from build123d import *

# Parameters (mm, degrees)
F0_R     = 0.635
F1_DEPTH = 2.54
F2_R     = 1.26999


# Not quite as in the source:
# - a fillet or chamfer is up to 0.001 mm smaller than in the source, because OpenCascade refuses the exact size


with BuildPart() as f1:
    # F0 (on Front) → F1 (new body)
    with BuildSketch(Plane.XZ):
        Polygon((15.0977487051, 33.894000689), (-8.7011743405, 33.894000689), (-8.7011743405, 30.6449289119), (-8.7011743405, 30.6394077664), (-8.7011743405, 28.5887729555), (-8.7011743405, 28.1049289119), (-8.7011743405, 23.0249289119), (21.375445649, 23.0249289119), (37.1712256595, 23.0249289119), (37.1712256595, 27.0205680281), (38.9492256595, 27.0205680281), (38.9492256595, 30.7752811804), (38.9492256595, 33.6518122062), (17.204430995, 33.6518122062), (17.204430995, 30.7752811804), (15.0977487051, 30.7752811804), align=None)
        with BuildLine():
            ThreePointArc((-6.7956986329, 25.5649289119), (-6.9816858268, 25.1159161058), (-7.4306986329, 24.9299289119))
            ThreePointArc((-7.4306986329, 24.9299289119), (-7.8797114389, 25.1159161058), (-8.0656986329, 25.5649289119))
            ThreePointArc((-8.0656986329, 25.5649289119), (-7.8797114389, 26.0139417179), (-7.4306986329, 26.1999289119))
            ThreePointArc((-7.4306986329, 26.1999289119), (-6.9816858268, 26.0139417179), (-6.7956986329, 25.5649289119))
        make_face(mode=Mode.SUBTRACT)
        with BuildLine():
            ThreePointArc((-7.4306986329, 28.7399289119), (-6.9816858268, 28.5539417179), (-6.7956986329, 28.1049289119))
            ThreePointArc((-6.7956986329, 28.1049289119), (-6.9816858268, 27.6559161058), (-7.4306986329, 27.4699289119))
            ThreePointArc((-7.4306986329, 27.4699289119), (-7.8797114389, 27.6559161058), (-8.0656986329, 28.1049289119))
            ThreePointArc((-8.0656986329, 28.1049289119), (-7.8797114389, 28.5539417179), (-7.4306986329, 28.7399289119))
        make_face(mode=Mode.SUBTRACT)
        with BuildLine():
            ThreePointArc((-7.4306986329, 30.0099289119), (-7.8797114389, 30.1959161058), (-8.0656986329, 30.6449289119))
            ThreePointArc((-8.0656986329, 30.6449289119), (-7.8797114389, 31.0939417179), (-7.4306986329, 31.2799289119))
            ThreePointArc((-7.4306986329, 31.2799289119), (-6.9816858268, 31.0939417179), (-6.7956986329, 30.6449289119))
            ThreePointArc((-6.7956986329, 30.6449289119), (-6.9816858268, 30.1959161058), (-7.4306986329, 30.0099289119))
        make_face(mode=Mode.SUBTRACT)
        with BuildLine():
            ThreePointArc((13.1927487051, 25.5649289119), (13.0067615112, 25.1159161058), (12.5577487051, 24.9299289119))
            ThreePointArc((12.5577487051, 24.9299289119), (11.9227487051, 25.5649289119), (12.5577487051, 26.1999289119))
            ThreePointArc((12.5577487051, 26.1999289119), (13.0067615112, 26.0139417179), (13.1927487051, 25.5649289119))
        make_face(mode=Mode.SUBTRACT)
        with BuildLine():
            ThreePointArc((12.5577487051, 28.7399289119), (13.0067615112, 28.5539417179), (13.1927487051, 28.1049289119))
            ThreePointArc((13.1927487051, 28.1049289119), (13.0067615112, 27.6559161058), (12.5577487051, 27.4699289119))
            ThreePointArc((12.5577487051, 27.4699289119), (11.9227487051, 28.1049289119), (12.5577487051, 28.7399289119))
        make_face(mode=Mode.SUBTRACT)
        with BuildLine():
            ThreePointArc((13.1927487051, 30.6449289119), (13.0067615112, 30.1959161058), (12.5577487051, 30.0099289119))
            ThreePointArc((12.5577487051, 30.0099289119), (11.9227487051, 30.6449289119), (12.5577487051, 31.2799289119))
            ThreePointArc((12.5577487051, 31.2799289119), (13.0067615112, 31.0939417179), (13.1927487051, 30.6449289119))
        make_face(mode=Mode.SUBTRACT)
        with Locations((19.744430995, 25.3227458062)):
            Circle(F0_R, mode=Mode.SUBTRACT)
        with Locations((19.744430995, 27.8627458062)):
            Circle(F0_R, mode=Mode.SUBTRACT)
        with Locations((19.744430995, 30.4027458062)):
            Circle(F0_R, mode=Mode.SUBTRACT)
        with BuildLine():
            Line((21.375445649, 23.0249289119), (-8.7011743405, 23.0249289119))
            Line((-8.7011743405, 23.0249289119), (14.6481524707, 7.6804661495))
            Line((14.6481524707, 7.6804661495), (4.3133735196, -8.0457365195))
            Line((4.3133735196, -8.0457365195), (4.3133735196, -53.9590548808))
            Line((4.3133735196, -53.9590548808), (21.375445649, -53.9590548808))
            Line((21.375445649, -53.9590548808), (21.375445649, -19.4510648049))
            ThreePointArc((21.375445649, -19.4510648049), (20.105445649, -18.1810648049), (21.375445649, -16.9110648049))
            Line((21.375445649, -16.9110648049), (21.375445649, 23.0249289119))
        make_face()
        with BuildLine():
            Line((37.1712256595, 23.0249289119), (21.375445649, 23.0249289119))
            Line((21.375445649, 23.0249289119), (21.375445649, -16.9110648049))
            ThreePointArc((21.375445649, -16.9110648049), (22.2734712611, -17.2830391928), (22.645445649, -18.1810648049))
            Line((22.645445649, -18.1810648049), (30.3538220114, -18.1810648049))
            Line((30.3538220114, -18.1810648049), (30.3538220114, -7.9758184713))
            Line((30.3538220114, -7.9758184713), (38.9492256595, -7.9758184713))
            Line((38.9492256595, -7.9758184713), (38.9492256595, 5.319000689))
            Line((38.9492256595, 5.319000689), (38.9492256595, 21.9405680281))
            Line((38.9492256595, 21.9405680281), (37.1712256595, 21.9405680281))
            Line((37.1712256595, 21.9405680281), (37.1712256595, 23.0249289119))
        make_face()
        Polygon((4.3133735196, -53.9590548808), (4.3133735196, -8.0457365195), (-20.8784960799, -46.3796427219), (-44.3256125721, -31.185070223), (-46.598433602, -34.7022139158), (-30.3224786203, -45.2199339734), (-30.3224786203, -53.9590548808), align=None)
        with BuildLine():
            Line((30.3538220114, -18.1810648049), (22.645445649, -18.1810648049))
            ThreePointArc((22.645445649, -18.1810648049), (22.2734712611, -19.079090417), (21.375445649, -19.4510648049))
            Line((21.375445649, -19.4510648049), (21.375445649, -53.9590548808))
            Line((21.375445649, -53.9590548808), (38.9492256595, -53.9590548808))
            Line((38.9492256595, -53.9590548808), (38.9492256595, -45.480999311))
            Line((38.9492256595, -45.480999311), (38.9492256595, -42.0136552247))
            Line((38.9492256595, -42.0136552247), (37.1712256595, -42.0136552247))
            Line((37.1712256595, -42.0136552247), (37.1712256595, -36.9336552247))
            Line((37.1712256595, -36.9336552247), (38.9492256595, -36.9336552247))
            Line((38.9492256595, -36.9336552247), (38.9492256595, -28.3863111384))
            Line((38.9492256595, -28.3863111384), (30.3538220114, -28.3863111384))
            Line((30.3538220114, -28.3863111384), (30.3538220114, -18.1810648049))
        make_face()
        Polygon((38.9492256595, -42.0136552247), (38.9492256595, -45.480999311), (38.9764610146, -42.0136552247), align=None)
        Polygon((39.0835013158, -28.3863111384), (38.9492256595, -28.3863111384), (38.9492256595, -36.9336552247), (39.0163634877, -36.9336552247), align=None)
    extrude(amount=F1_DEPTH)

    # F2 (radius 1.27 in the source; OpenCascade refuses exactly that, so slightly less here)
    f2_edges = [f1.edges().sort_by_distance(p)[0] for p in [
        (20.105446, -2.54, -18.181065),
        (20.105446, 0, -18.181065),
    ]]
    fillet(f2_edges, radius=F2_R)


solid = f1.part
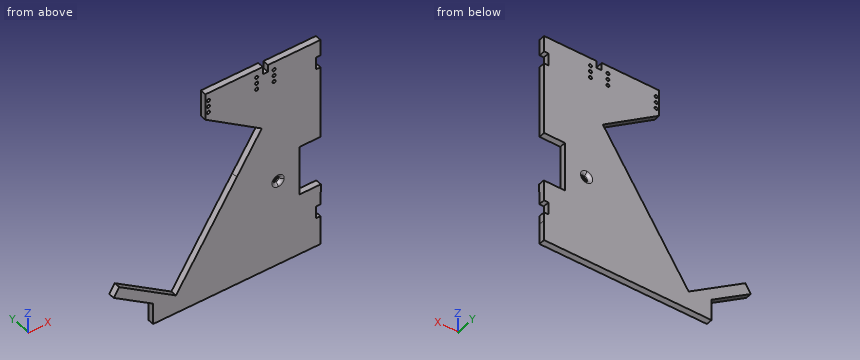
Part model, mm, in its own coordinate system. Coordinates: 2 decimals unless noted, no trailing zeros. Order: outer loops, then holes, each group sorted by start corner. A loop starts at its lowest first (then second) coordinate and runs counter-clockwise, first axis right, second up. Notation, with made-up numbers: M 44.25,3.5 L 103.25,3.5 A33 cw 103.25,36.5 Z; hole C -40,-15 d4. An arc over 180 degrees is marked long. One line per question, with ' | ' between items.
Q1. Slice it at D-D (z = 12). Give the cut face in (x, y).
A:
outline: M 8.08,-2.54 L 38.95,-2.54 L 38.95,0 L 8.08,0 Z
Q2. Pin check, flat tips, straight feed: P1, Ø1, axis at x = 19.74, z = 27.86, coming from the +Y side; P2, Ø0.8, axis at y = -1, z = -40, coming from the +X side; P3, Ø1.3, axis at y = -1.5, z = 32.5, coming from the +X side; P4, Ø0.8, axis at x = 34, y = -1.5, coming from the +Z side. Stop position of each tip, or through.
A:
P1: passes through | P2: stops at x = 37.17 | P3: stops at x = 38.95 | P4: stops at z = 33.65
Q3. Drill centre lines: line 1 (Z direction, x = 12, y = -1.8); line 2 (X direction, y = -1.45, z = 25); line 3 (Z direction, x = -18, y = -1.4). Where is each one in solid material? Low to high.
A:
line 1: z = -53.96 to 3.65, 9.42 to 25.26, 25.87 to 27.8, 28.41 to 30.34, 30.95 to 33.89 | line 2: x = -8.7 to -7.72, -7.14 to 12.27, 12.85 to 19.2, 20.29 to 37.17 | line 3: z = -53.96 to -42
Q4. Slice it at A-A (x = 2.5). Give the cut face in (y, z), and give its area (3 significant figures).
A:
outline: M -2.54,-53.96 L 0,-53.96 L 0,-10.81 L -2.54,-10.81 Z; M -2.54,15.66 L 0,15.66 L 0,33.89 L -2.54,33.89 Z | area: 156 mm^2
Q5. Slice it at B-B (z = -40). Give the cut face in (x, y).
A:
outline: M -38.4,-2.54 L -30.72,-2.54 L -30.72,0 L -38.4,0 Z; M -16.69,-2.54 L 37.17,-2.54 L 37.17,0 L -16.69,0 Z
Q6. Slice it at C-C (y = -2.1). Count the separate pieces of the cut face and the enclosed holes in it, and give its area (3 significant figures).
A:
separate pieces: 1 | enclosed holes: 10 | area: 3,750 mm^2
